Here's how the part is built. I have some questions about the finished solid (model axes, mm). A direction names the side the tool comes from. Give positions to 0.01 mm unless a question says otherwise; leave off trailing zeros. Loops run counter-clockwise (first coordinate to the right, second up) from the corner with the lowest first, then second, coordinate; pieces in that order, holes last. Notation, with made-up numbers: (14.25, 56.25) - (25.25, 56.25) arc R28 ccw to (25.25, 90.25) - close; hole circle Ø11 at (66.25, -32). An arc over 180 degrees is marked (long way). One line per item, written item: value. Start each with the question number.
```python
from build123d import *

# Parameters (mm, degrees)
SKETCH1_W           = 103
SKETCH1_H           = 153
BOSS_EXTRUDE1_DEPTH = 60
SHELL1_T            = -1.5
CUT_EXTRUDE1_REACH  = 174.224
SKETCH2_R           = 14
SKETCH3_W           = 58.5
SKETCH3_H           = 1.5
BOSS_EXTRUDE2_DEPTH = 15
CUT_EXTRUDE2_REACH  = 112.02
SKETCH4_R           = 3


with BuildPart() as part:
    # Sketch1 → Boss-Extrude1 (new body)
    with BuildSketch(Plane.XY):
        Rectangle(SKETCH1_W, SKETCH1_H)
    extrude(amount=BOSS_EXTRUDE1_DEPTH)

    # Shell1
    shell1_openings = [part.faces().sort_by_distance(p)[0] for p in [
        (0, 0, 60),
        (0, 76.5, 30),
    ]]
    offset(amount=SHELL1_T, openings=shell1_openings, kind=Kind.INTERSECTION)

    # Sketch2 → Cut-Extrude1 (cut, up to next)
    with BuildSketch(Plane.XZ.offset(76.5), mode=Mode.PRIVATE) as cut_extrude1_sk1:
        with Locations(Location((0, 30, 0), (0, 0, 270))):
            Circle(SKETCH2_R)
    cut_extrude1_tool1 = extrude(cut_extrude1_sk1.sketch, amount=-CUT_EXTRUDE1_REACH, mode=Mode.PRIVATE) & part.part
    add(cut_extrude1_tool1.solids().sort_by_distance((0, -76.5, 30))[0], mode=Mode.SUBTRACT)

    # Sketch3 → Boss-Extrude2 (add)
    with BuildSketch(Plane.ZY.offset(-50)):
        with Locations((30.75, 75.75)):
            Rectangle(SKETCH3_W, SKETCH3_H)
    boss_extrude2 = extrude(amount=BOSS_EXTRUDE2_DEPTH)

    # Mirror1: Boss-Extrude2 across plane
    add(boss_extrude2.mirror(Plane(origin=(0, 0, 0), x_dir=(0, 0, 1), z_dir=(1, 0, 0))))

    # Sketch4 → Cut-Extrude2 (cut, up to next)
    with BuildSketch(Plane(origin=(0, 0, 0), x_dir=(-1, 0, 0), z_dir=(0, 0, -1)), mode=Mode.PRIVATE) as cut_extrude2_sk1:
        with Locations((-30, 0)):
            Circle(SKETCH4_R)
    cut_extrude2_tool1 = extrude(cut_extrude2_sk1.sketch, amount=-CUT_EXTRUDE2_REACH, mode=Mode.PRIVATE) & part.part
    # Sketch4 → Cut-Extrude2 (cut, up to next)
    with BuildSketch(Plane(origin=(0, 0, 0), x_dir=(-1, 0, 0), z_dir=(0, 0, -1)), mode=Mode.PRIVATE) as cut_extrude2_sk2:
        with Locations(Location((30, 0, 0), (0, 0, 180))):
            Circle(SKETCH4_R)
    cut_extrude2_tool2 = extrude(cut_extrude2_sk2.sketch, amount=-CUT_EXTRUDE2_REACH, mode=Mode.PRIVATE) & part.part
    add(cut_extrude2_tool1.solids().sort_by_distance((30, 0, 0))[0], mode=Mode.SUBTRACT)
    add(cut_extrude2_tool2.solids().sort_by_distance((-30, 0, 0))[0], mode=Mode.SUBTRACT)


solid = part.part
```
(1) Will these pins go through, and if not, where does the flat tip stop? pin 1 (22.5 mm diameter, centred on x = 0, z = 30, fed in from -Y); pin 2 (1 mm diameter, centred on x = -9, z = 45, fed in from +Y); pin 3 (1.5 mm diameter, centred on x = -13.5, y = -18, fed in from +Z).
(2) If we section it at B-B on x = -30: List the corners of the cut face in (y, z) for me, plus the area to 3 significant figures.
(3) If we section it at A-A on y = 0: List the corners of the cut face in (x, z) for me.
(4) If we mould it in two halves opening along X, with no side actions, what happens to faces 1 (the face through (-12, -75, 17)), 2 (the face through (-51.5, -1, 30)), 3 (the face through (4, 76.5, 1))? For each: pulls with the +X half, pulls with the -X half, needs draft (parallel to the pull), parting line crosses it, or undercut.
(5) If we section it at D-D on y = 40: List the corners of the cut face in (x, z) for me, plus the area to 3 significant figures.
(6) Please list where these lines run through material, in increasing order: probe 1 along X at (y, z) = (-75.25, 30); probe 2 along Y at (x, z) = (-36, 6.5); probe 3 along X at (y, z) = (63.5, 22). Write a range as from..to.
(7) If we section it at C-C on z = 11.5: List the corners of the cut face in (x, y) for me.
(8) For faces 4 (the face through (-50, -1, 30)), 5 (the face through (0.616, -75.76, 43.986)), which set-ups out of +Z, -Z, +X, -X, +Y, -Y let a thin tool reach every point of the face, with its end or its side?
Found:
1. pin 1: through
1. pin 2: y = -75
1. pin 3: z = 1.5
2. outline: (-76.5, 0) - (-3, 0) - (-3, 1.5) - (-75, 1.5) - (-75, 60) - (-76.5, 60) - close; (3, 0) - (76.5, 0) - (76.5, 1.5) - (3, 1.5) - close
2. area: 308 mm^2
3. outline: (-51.5, 0) - (-33, 0) - (-33, 1.5) - (-50, 1.5) - (-50, 60) - (-51.5, 60) - close; (-27, 0) - (27, 0) - (27, 1.5) - (-27, 1.5) - close; (33, 0) - (51.5, 0) - (51.5, 60) - (50, 60) - (50, 1.5) - (33, 1.5) - close
4. face 1: undercut
4. face 2: pulls with the -X half
4. face 3: needs draft
5. outline: (-51.5, 0) - (51.5, 0) - (51.5, 60) - (50, 60) - (50, 1.5) - (-50, 1.5) - (-50, 60) - (-51.5, 60) - close
5. area: 330 mm^2
6. probe 1: -51.5..-14, 14..51.5
6. probe 2: -76.5..-75, 75..76.5
6. probe 3: -51.5..-50, 50..51.5
7. outline: (-51.5, -76.5) - (51.5, -76.5) - (51.5, 76.5) - (35, 76.5) - (35, 75) - (50, 75) - (50, -75) - (-50, -75) - (-50, 75) - (-35, 75) - (-35, 76.5) - (-51.5, 76.5) - close
8. face 4: +Z
8. face 5: +Y, -Y
